Can you work these out from the model? Positions are in its coordinate system, mm. Coordinates: 2 decimals unless noted, no trailing zeros. Order: outer loops, then holes, each group sorted by start corner. A loop starts at its lowest first (then second) coordinate and runs counter-clockwise, first axis right, second up. Notation, with made-up numbers: (64.25, 55) - (120.25, 55) arc R19 cw to (120.25, 88) - close; hole circle Ø6 at (1.5, 10). An arc over 180 degrees is marked (long way). Use a Markdown table: item, result. Add a question column.
(1) I want a section at D-D (y = 0.4). State how many separate pieces and enclosed holes the cut face has, and give its area (3 significant figures).
(2) We'd pull the mould along Z, two halves only. Please class faces 1 (the cylindrical face through (0, 1, 27)), 2 (the flat face through (0, 0, 0)): pulls with the +Z half, pulls with the -Z half, needs draft (parallel to the pull), parting line crosses it, or undercut.
(3) I want a section at B-B (x = -31). List the corners of the cut face in (y, z) for me.
(4) If I drill on L1, parallel to X at y = 1.9, z = 0; L2, parallel to Z at x = 0, y = 1.7; L3, parallel to X at y = 1.7, z = 30.5, over which ranges is the centre line in solid material (lowest first)? Write a range as [from, to].
(5) For pin 1 Ø4 at (x, z) = (0, -30.5) entering from +Y; pin 2 Ø1 at (x, y) = (-17, 1.5) entering from -Z; pin 3 Ø1.5 at (y, z) = (1.5, -40.5) entering from -X; pin 4 Ø1.2 at (y, z) = (1, 51) entering from +X, each with a flat end and sliding along its axis, tell me the tip position at first contact or that it passes through.
(6) I want a section at A-A (z = -30.5). List the corners of the cut face in (x, y) for me.
(7) I want a section at C-C (z = 0). List the corners of the cut face in (x, y) for me.
```python
from build123d import *

# Parameters (mm, degrees)
SKETCH_1_R      = 3.5
EXTRUDE_1_DEPTH = 2.5
FILLET_1_R      = 2


with BuildPart() as part:
    # 草图1 → 凸台-拉伸1 (new body)
    with BuildSketch(Plane(origin=(0, 0, 0), x_dir=(1, 0, 0), z_dir=(0, 1, 0))):
        Polygon((-13, 72), (13, 72), (13, 13), (42.5, 13), (42.5, -13), (13, -13), (13, -72), (-13, -72), (-13, -13), (-42.5, -13), (-42.5, 13), (-13, 13), align=None)
        with Locations((0, -60.5)):
            Circle(SKETCH_1_R, mode=Mode.SUBTRACT)
        with Locations((0, -30.5)):
            Circle(SKETCH_1_R, mode=Mode.SUBTRACT)
        with Locations((-31, 0)):
            Circle(SKETCH_1_R, mode=Mode.SUBTRACT)
        with Locations((31, 0)):
            Circle(SKETCH_1_R, mode=Mode.SUBTRACT)
        with Locations((0, 60.5)):
            Circle(SKETCH_1_R, mode=Mode.SUBTRACT)
        with Locations((0, 30.5)):
            Circle(SKETCH_1_R, mode=Mode.SUBTRACT)
    extrude(amount=EXTRUDE_1_DEPTH)

    # 圆角1
    fillet_1_edges = [part.edges().sort_by_distance(p)[0] for p in [
        (13, 1.25, 72),
        (-13, 1.25, 72),
        (-13, 1.25, 13),
        (-42.5, 1.25, 13),
        (-42.5, 1.25, -13),
        (-13, 1.25, -13),
        (-13, 1.25, -72),
        (13, 1.25, -72),
        (13, 1.25, -13),
        (42.5, 1.25, -13),
        (42.5, 1.25, 13),
        (13, 1.25, 13),
    ]]
    fillet(fillet_1_edges, radius=FILLET_1_R)


solid = part.part
```
Answers follow:
| question | item | result |
|---|---|---|
| 1 | separate pieces | 1 |
| 1 | enclosed holes | 6 |
| 1 | area | 5,040 mm² |
| 2 | face 1 | undercut |
| 2 | face 2 | needs draft |
| 3 | outline | (0, -13) - (2.5, -13) - (2.5, -3.5) - (0, -3.5) - close; (0, 3.5) - (2.5, 3.5) - (2.5, 13) - (0, 13) - close |
| 4 | L1 | x = [-42.5, -34.5], [-27.5, 27.5], [34.5, 42.5] |
| 4 | L2 | z = [-72, -64], [-57, -34], [-27, 27], [34, 57], [64, 72] |
| 4 | L3 | x = [-13, -3.5], [3.5, 13] |
| 5 | pin 1 | passes through |
| 5 | pin 2 | stops at z = -13 |
| 5 | pin 3 | stops at x = -13 |
| 5 | pin 4 | stops at x = 13 |
| 6 | outline | (-13, 0) - (-3.5, 0) - (-3.5, 2.5) - (-13, 2.5) - close; (3.5, 0) - (13, 0) - (13, 2.5) - (3.5, 2.5) - close |
| 7 | outline | (-42.5, 0) - (-34.5, 0) - (-34.5, 2.5) - (-42.5, 2.5) - close; (-27.5, 0) - (27.5, 0) - (27.5, 2.5) - (-27.5, 2.5) - close; (34.5, 0) - (42.5, 0) - (42.5, 2.5) - (34.5, 2.5) - close |
